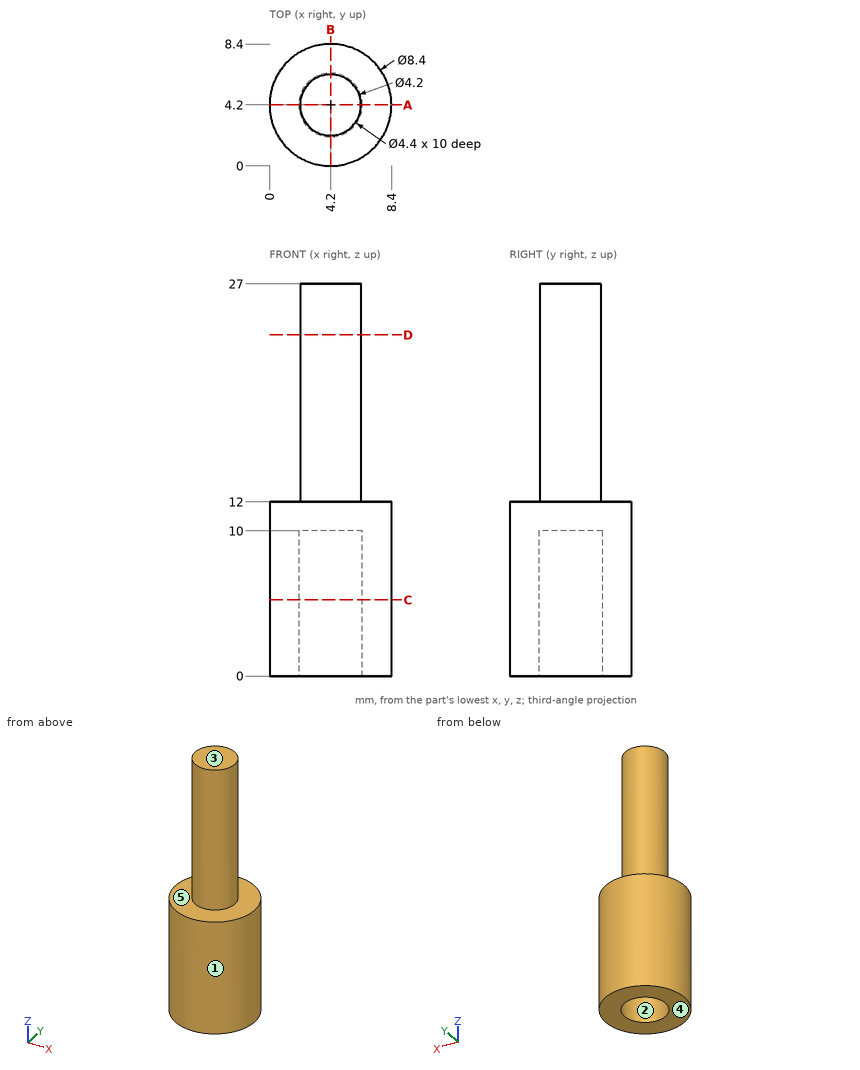
Geometry: see drawing. Coordinates: mm, zero at the bounding-box minimum. A direction names the side the tool comes from. Coordinates: 2 decimals unless noted, no trailing zeros. Loops run counter-clockwise (first coordinate to the right, second up) from the corner with the lowest first, then second, coordinate; pieces in that order, holes last. Notation, with made-up numbers: (9, 80) - (27, 80) arc R11 ccw to (27, 88) - close; hole circle Ø11 at (18.5, -4.75). An arc over 180 degrees is marked (long way). Put each result on its own line as item: value. Start each with the question number.
Q1. Line query: line 1 (Y direction, x = 4.2, z = 7.75); line 2 (X direction, y = 5.5, z = 7.5); line 3 (Z direction, x = 8, y = 5.75). Output: solid intervals per line, ascending.
Q2. Pin query (flat end, axial travel): pin 1 Ø1.5 at (y, z) = (2, 15) entering from +X; pin 2 Ø5 at (x, z) = (6, 18.5) entering from -Y; pin 3 Ø1.3 at (x, y) = (4.5, 3) entering from -Z. Return the tip coordinate at first contact, or that it passes through.
Q3. Cut plane A-A, the plane y = 4.2. Return loops of the section in (x, z).
Q4. Cut plane C-C, the plane z = 5.25. Return loops of the section in (x, y), and give its area (3 significant figures).
Q5. Pull-direction query (X, two-part tool) for the marked faces 1, 2 and 3; classes: released by +X, released by -X, zero draft, split by the parting line, or undercut.
Q6. Set-up query: the marked faces 4 and 5. Return all of +Z, -Z, +X, -X, +Y, -Y with unobstructed straight access to the full face (end or side cutting, diameter ignored); none if empty.
Q7. Cut plane D-D, the plane z = 23.5. Return loops of the section in (x, y).
Filled sheet:
1. line 1: 0 to 2, 6.4 to 8.4
1. line 2: 0.21 to 2.43, 5.97 to 8.19
1. line 3: 0 to 12
2. pin 1: x = 5.72
2. pin 2: y = 2.1
2. pin 3: z = 10
3. outline: (0, 0) - (2, 0) - (2, 10) - (6.4, 10) - (6.4, 0) - (8.4, 0) - (8.4, 12) - (6.3, 12) - (6.3, 27) - (2.1, 27) - (2.1, 12) - (0, 12) - close
4. outline: circle Ø8.4 at (4.2, 4.2); hole circle Ø4.4 at (4.2, 4.2)
4. area: 40.2 mm²
5. face 1: split by the parting line
5. face 2: undercut
5. face 3: zero draft
6. face 4: -Z, +X, -X, +Y, -Y
6. face 5: +Z
7. outline: circle Ø4.2 at (4.2, 4.2)
